from build123d import *

# Parameters (mm, degrees)
SKETCH1_R           = 75
BOSS_EXTRUDE1_DEPTH = 2
SKETCH2_R           = 70
BOSS_EXTRUDE2_DEPTH = 6
SKETCH3_R           = 75
BOSS_EXTRUDE3_DEPTH = 2
CHAMFER1_SIZE       = 1
CHAMFER2_SIZE       = 1
SKETCH4_R           = 20
BOSS_EXTRUDE5_DEPTH = 20
SKETCH5_R           = 4.5
CUT_EXTRUDE1_DEPTH  = 111.227038425
CUT_EXTRUDE2_START  = -5
SKETCH6_W           = 3
SKETCH6_H           = 6
CUT_EXTRUDE2_DEPTH  = 20


with BuildPart() as part:
    # Sketch1 → Boss-Extrude1 (new body)
    with BuildSketch(Plane.XY):
        Circle(SKETCH1_R)
    extrude(amount=BOSS_EXTRUDE1_DEPTH)

    # Sketch2 → Boss-Extrude2 (add)
    with BuildSketch(Plane.XY.offset(2)):
        Circle(SKETCH2_R)
    extrude(amount=BOSS_EXTRUDE2_DEPTH)

    # Sketch3 → Boss-Extrude3 (add)
    with BuildSketch(Plane.XY.offset(8)):
        Circle(SKETCH3_R)
    extrude(amount=BOSS_EXTRUDE3_DEPTH)

    # Chamfer1
    chamfer1_edges = [part.edges().sort_by_distance(p)[0] for p in [
        (-75, 0, 0),
        (-75, 0, 2),
        (-70, 0, 2),
    ]]
    chamfer(chamfer1_edges, length=CHAMFER1_SIZE - 0.0001)  # a hair under: the kernel refuses the full size

    # Chamfer2
    chamfer2_edges = [part.edges().sort_by_distance(p)[0] for p in [
        (-75, 0, 8),
        (-75, 0, 10),
        (-70, 0, 8),
    ]]
    chamfer(chamfer2_edges, length=CHAMFER2_SIZE - 0.0001)  # a hair under: the kernel refuses the full size

    # Sketch4 → Boss-Extrude5 (add)
    with BuildSketch(Plane.XY.offset(10)):
        Circle(SKETCH4_R)
    extrude(amount=BOSS_EXTRUDE5_DEPTH)

    # Sketch5 → Cut-Extrude1 (cut, through all)
    with BuildSketch(Plane.XY.offset(30)):
        Circle(SKETCH5_R)
    extrude(amount=-CUT_EXTRUDE1_DEPTH, mode=Mode.SUBTRACT)

    # Sketch6 → Cut-Extrude2 (cut)
    with BuildSketch(Plane.XY.offset(30).offset(CUT_EXTRUDE2_START)):
        with Locations((0, 4.5)):
            Rectangle(SKETCH6_W, SKETCH6_H)
    extrude(amount=-CUT_EXTRUDE2_DEPTH, mode=Mode.SUBTRACT)


solid = part.part
Verification items for the finished model (mm, model axes). A direction names the side the tool comes from. Give positions to 0.01 mm unless a question says otherwise; leave off trailing zeros. Loops run counter-clockwise (first coordinate to the right, second up) from the corner with the lowest first, then second, coordinate; pieces in that order, holes last. Notation, with made-up numbers: (88.5, 58) - (128.5, 58) arc R31 ccw to (128.5, 96) - close; hole circle Ø3 at (35, 81). An arc over 180 degrees is marked (long way). Write item = value, one per line. Start each with the question number.
Q1. Mould release check, pull along Y, two halves, no side actions. Record for faces 1 (the face through (15, 1, 0)), 2 (the face through (-1.5, 6, 15)), 3 (the face through (-55.55, -42.594, 4.972)): released by +Y, released by -Y, zero draft, split by the parting line, or undercut.
Q2. Tool access check on faces 4 (the face through (-0.98, -4.39, 15.21)), 5 (the face through (-66, 28, 2)), 6 (the face through (15, -15, 10)). Record the directions out of +Z, -Z, +X, -X, +Y, -Y that give a thin tool (end or side, any length) a straight path to the whole face; none if there is none.
Q3. Thickness scan on line 1 (Y direction, x = 0, z = 17); line 2 (Z direction, x = 54.5, y = 11.5); line 3 (Y direction, x = 67, z = 8.25). Record the ranges inside material, lowest first.
Q4. Depth check by flat-ended pin: P1, Ø5, axis at y = 59.5, z = 7, coming from the -X side; P2, Ø12, axis at y = 22.5, z = 20.5, coming from the +X side; P3, Ø1, axis at x = -35, y = 46, coming from the +Z side. Enter the tip coordinate at first touch or a pass-through.
Q5. Cross-section at B-B, the plane z = 19. Enter the section's corners in (x, y), and give its area (3 significant figures).
Answer key:
q1.face_1 = zero draft
q1.face_2 = undercut
q1.face_3 = split by the parting line
q2.face_4 = +Z, -Z
q2.face_5 = none
q2.face_6 = +Z
q3.line_1 = -20 to -4.5, 7.5 to 20
q3.line_2 = 0 to 10
q3.line_3 = -32 to 32
q4.P1 = -47.55
q4.P2 = 11.3
q4.P3 = 10
q5.outline = circle Ø40 at (0, 0); hole (-1.5, 4.24) arc R4.5 ccw (long way) to (1.5, 4.24) - (1.5, 7.5) - (-1.5, 7.5) - close
q5.area = 1,180 mm^2
